Work out the finished part from the listing and answer in its coordinate system (mm). A direction names the side the tool comes from. Coordinates: 2 decimals unless noted, no trailing zeros. Answer as CSV lines item,"result". Start each with the question number.
Item 1: For a pull along Z with two mould halves and no side action, classify faces 4 (the face through (70.61, 2.01, -12.04)), 5 (the face through (2.51, -0.74, -42.65)), 6 (the face through (77.994, -0.6, -6.5)), 7 (the face through (77.07, 0.49, -2.9)) as pulls with the +Z half, pulls with the -Z half, needs draft (parallel to the pull), parting line crosses it, or undercut.
Item 2: Each of these flat-tipped pins is pushed along its axis until it touches: pin 1 Ø0.8 at (x, y) = (52.5, 0.5) entering from -Z; pin 2 Ø1.6 at (y, z) = (-0.5, -43) entering from -X; pin 3 Ø1.2 at (y, z) = (-1, -42.5) entering from +X. Where does it stop, or does it pass through?
Item 3: Which of the six approach directions +Z, -Z, +X, -X, +Y, -Y give full straight-line access (tool end or side, diameter ignored) to faces 1 (the face through (2.9, 0.49, -2.93)), 2 (the face through (72, 2, -20.5)), 3 (the face through (79, 1, -24))?
Item 4: Straight lines are drawn through the part: L1, parallel to Z at x = 28, y = 1.5; L2, parallel to Y at x = 69, z = -16; L3, parallel to X at y = -0.45, z = -24. For each, find the intervals that lie inside material, in ascending order.
Item 5: Section C-C (z = -25.5) is taken. Count the separate pieces of the cut face and the enclosed holes in it, then the cut area to 3 significant figures.
Autodesk Inventor part; units mm, degrees
ref_plane "Pracovní rovina1" through (77, 0, -24.5) normal (0, 0, -1) x (-1, 0, 0)
ref_plane "YZ Plane" through (0, 0, 0) normal (1, 0, 0) x (0, 1, 0)
ref_plane "XZ Plane" through (0, 0, 0) normal (0, 1, 0) x (-1, 0, 0)
sketch "Náčrt1" plane through (0, 0, 0) normal (0, 1, 0) x (-1, 0, 0)
  line L0 (0, 0) -> (-80, 0)
  line L1 (-80, 0) -> (-80, -49)
  line L2 (-80, -49) -> (0, -49)
  line L3 (0, -49) -> (0, 0)
  dimension "d0" = 80
  dimension "d1" = 49
extrude "Vysunutí1" add sketch "Náčrt1" along normal blind 3
chamfer "Zkosení1" distance 3 angle 45 4 edges at (0, 1.5, 0) (0, 1.5, -49) (80, 1.5, -49) (80, 1.5, 0)
chamfer "Zkosení2" distance 3 angle 45 4 edges at (40, 3, 0) (0, 3, -24.5) (40, 3, -49) (80, 3, -24.5)
sketch "Náčrt2" plane through (0, 3, 0) normal (0, 1, 0) x (1, 0, 0)
  line L0 (18, 41.5) -> (62, 41.5)
  line L1 (62, 41.5) -> (62, 7.5)
  line L2 (62, 7.5) -> (18, 7.5)
  line L3 (18, 7.5) -> (18, 41.5)
  line L4 (77, 49) -> (3, 49)
  line L5 (0, 46) -> (0, 3)
  point P0 (0, 0)
  dimension "d11" = 44
  dimension "d12" = 34
  dimension "d13" = 7.5
  dimension "d14" = 18
extrude "Vysunutí2" cut sketch "Náčrt2" against normal blind 2.5
sketch "Náčrt3" plane through (0, 3, 0) normal (0, 1, 0) x (1, 0, 0)
  line L0 (63, 42.5) -> (17, 42.5)
  line L1 (17, 42.5) -> (17, 6.5)
  line L2 (17, 6.5) -> (63, 6.5)
  line L3 (63, 6.5) -> (63, 42.5)
  line L4 (63, 42.5) -> (17, 6.5) construction
  line L5 (17, 42.5) -> (63, 6.5) construction
  point P0 (0, 0)
  point P1 (40, 24.5)
  dimension "d17" = 46
  dimension "d18" = 36
extrude "Vysunutí3" cut sketch "Náčrt3" against normal blind 1
sketch "Náčrt4" plane through (0, 3, 0) normal (0, 1, 0) x (1, 0, 0)
  line L0 (75.5, 16) -> (69, 16)
  line L1 (69, 16) -> (72.25, 8)
  line L2 (75.5, 16) -> (72.25, 8)
  line L3 (3, 0) -> (77, 0)
  line L4 (0, 46) -> (0, 3)
  point P0 (0, 0)
  dimension "d21" = 6.5
extrude "Vysunutí4" cut sketch "Náčrt4" against normal blind 2.5
chamfer "Zkosení3" distance 1 angle 45 3 edges at (69, 1.75, -16) (75.5, 1.75, -16) (72.25, 1.75, -8)
ref_plane "Pracovní rovina1" through (77, 0, -24.5) normal (0, 0, -1) x (-1, 0, 0)
mirror "Zrcadlit1" about plane through (77, 0, -24.5) normal (0, 0, -1) of "Vysunutí4", "Zkosení3"
sketch "Náčrt5" plane through (0, 3, 0) normal (0, 1, 0) x (1, 0, 0)
  line L0 (69.3705, 20.5) -> (74.8705, 20.5)
  line L1 (74.8705, 20.5) -> (74.8705, 28.5)
  line L2 (74.8705, 28.5) -> (69.3705, 28.5)
  line L3 (69.3705, 28.5) -> (69.3705, 20.5)
  line L4 (3, 0) -> (77, 0)
  point P0 (0, 0)
  dimension "d30" = 5.5
  dimension "d31" = 8
  dimension "d32" = 20.5
extrude "Vysunutí5" cut sketch "Náčrt5" against normal blind 2.5
chamfer "Zkosení4" distance 1 angle 45 4 edges at (69.3705, 1.75, -28.5) (69.3705, 1.75, -20.5) (74.8705, 1.75, -20.5) (74.8705, 1.75, -28.5)
sketch "Náčrt6" plane through (0, 3, 0) normal (0, 1, 0) x (1, 0, 0)
  point P0 (0, 0)
sketch "Náčrt7" plane through (0, 0, 0) normal (0, -1, 0) x (1, 0, 0)
  line L0 (3.8284, -2) -> (76.1716, -2)
  line L1 (77.9939, -3.8223) -> (77.9939, -45.1777)
  line L2 (76.2085, -46.9631) -> (3.9251, -46.9631)
  line L3 (2, -46) -> (2, -3.8284)
  line L4 (3, 0) -> (77, 0)
  line L5 (0, -46) -> (0, -3)
  line L6 (0, -46) -> (2.8284, -46) construction
  line L7 (2, -45.0688) -> (3.9251, -46.9631)
  line L8 (3, -49) -> (0, -46)
  line L9 (80, -46) -> (77, -49)
  line L10 (80, -46) -> (82.8284, -46) construction
  line L11 (77.9939, -45.1777) -> (76.2085, -46.9631)
  line L12 (77, 0) -> (80, -3)
  line L13 (76.1716, -2) -> (77.9939, -3.8223)
  line L14 (2, -3.8284) -> (3.8284, -2)
  line L15 (0, -3) -> (3, 0)
  point P0 (0, 0)
  dimension "d40" = 2
  dimension "d41" = 2
  dimension "d43" = 2
  dimension "d45" = 2
  dimension "d46" = 2
  dimension "d47" = 2
extrude "Vysunutí6" cut sketch "Náčrt7" against normal blind 1
sketch "Náčrt8" plane through (77.9939, 0, -45.1777) normal (-1, 0, 0) x (0, 0, 1)
  line L0 (1.7879, 1) -> (1.7879, -1.5)
  line L1 (1.7879, -1.5) -> (39.5674, -1.5)
  line L2 (39.5674, -1.5) -> (39.5674, 1)
  line L3 (41.3554, 1) -> (0, 1)
  line L4 (39.5674, 1) -> (1.7879, 1)
  point P0 (45.1777, 0)
extrude "Vysunutí7" add sketch "Náčrt8" along normal blind 1
chamfer "Zkosení5" distance 1.5 angle 45 2 edges at (77.4939, -1.5, -5.6103) (77.4939, -1.5, -43.3897)
sketch "Náčrt9" plane through (77.9939, 0, -45.1777) normal (1, 0, 0) x (0, 0, -1)
  line L0 (-3.2879, -1.5) -> (-3.2879, 0)
  line L1 (-3.2879, -1.5) -> (-38.0674, -1.5)
  line L2 (-3.2879, -1.5) -> (-38.0674, -1.5)
  line L3 (-38.0674, -1.5) -> (-38.0674, 0)
  line L4 (-42.1777, 0) -> (0.8223, 0)
  point P0 (-45.1777, 0)
  point P1 (-1.7879, 0)
extrude "Vysunutí8" add sketch "Náčrt9" along normal blind 0.5 draft -80
ref_plane "Pracovní rovina2" through (39.9969, 0, -45.1777) normal (-1, 0, 0) x (0, 0, 1)
mirror "Zrcadlit2" about plane through (39.9969, 0, -45.1777) normal (-1, 0, 0) of "Vysunutí7", "Zkosení5", "Vysunutí8"
properties part number "TopCover"
Checked values:
1,face 4,"undercut"
1,face 5,"pulls with the -Z half"
1,face 6,"needs draft"
1,face 7,"undercut"
2,pin 1,"stops at z = -48.9"
2,pin 2,"stops at x = 0"
2,pin 3,"stops at x = 77.99"
3,face 1,"-Y"
3,face 2,"+Y, -Y"
3,face 3,"+Z, -Z, +X, +Y"
4,L1,"z = -47.5 to -41.5, -7.5 to -1.5"
4,L2,"y = 1 to 3"
4,L3,"x = 1.92 to 3, 76.99 to 78.07"
5,separate pieces,"3"
5,enclosed holes,"0"
5,area,"59.2 mm^2"
